Autodesk Fusion 360 part; units mm, degrees
sketch "草图1" plane through (0, 0, 0) normal (0, 0, 1) x (1, 0, 0)
  circle A0 centre (0, 0) radius 10
  circle A1 centre (0, 0) radius 7 construction
  line L0 (-4, 0) -> (3, 0)
  circle A2 centre (7, 0) radius 1.6
  circle A3 centre (0, 7) radius 1.6
  circle A4 centre (-7, 0) radius 1.6
  circle A5 centre (0, -7) radius 1.6
  dimension "d1" = 20
  dimension "d2" = 14
  dimension "d3" = 3.2
  dimension "d5" = 360
extrude "拉伸1" add sketch "草图1" along normal blind 2 makes body 1
sketch "草图2" plane through (0, 0, 2) normal (0, 0, 1) x (-1, 0, 0)
  circle A0 centre (0, 7) radius 1.6
  circle A1 centre (7, 0) radius 1.6
  circle A2 centre (-7, 0) radius 1.6
  circle A3 centre (0, -7) radius 1.6
  circle A4 centre (0, 0) radius 10
  circle A5 centre (0, 0) radius 4.5
  dimension "d8" = 9
extrude "拉伸2" add sketch "草图2" along normal blind 2.5 contours A5 bodies 1
sketch "草图3" plane through (0, 0, 4.5) normal (0, 0, 1) x (-1, 0, 0)
  circle A0 centre (0, 0) radius 4.5
  circle A1 centre (0, 0) radius 2.75
  dimension "d11" = 5.5
extrude "拉伸3" cut sketch "草图3" against normal blind 4 contours A1 bodies 1
sketch "草图4" plane through (0, 0, 0.5) normal (0, 0, 1) x (-1, 0, 0)
  circle A0 centre (0, 0) radius 2.75
  circle A1 centre (0, 0) radius 1.6
  dimension "d14" = 3.2
extrude "拉伸4" cut sketch "草图4" against normal blind 2 contours A1 bodies 1
copy_body "实体->零部件1" bodies 1 removing the originals makes body 2 in component "Component'"
component "Component'" placed x (1, 0, 0) y (0, 1, 0) z (0, 0, 1) at (0, 0, 0)
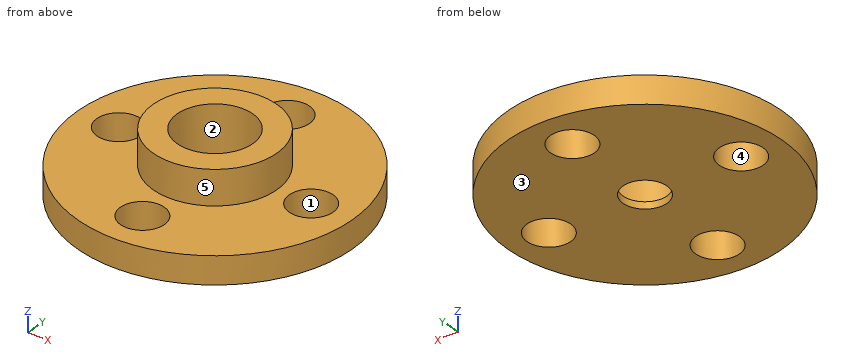
Design review of the part built by this model. Coordinates are the model's own, in mm. Face numbers are marked on the shaded views. A direction names the side the tool comes from. Give positions to 0.01 mm unless a question says otherwise; leave off trailing zeros. Order: outer loops, then holes, each group sorted by start corner. A loop starts at its lowest first (then second) coordinate and runs counter-clockwise, first axis right, second up. Notation, with made-up numbers: (45, 75) - (56, 75) arc R20 ccw to (56, 113) - close; hole circle Ø8 at (51.5, 31). An arc over 180 degrees is marked (long way). Write item = value, one per line. Start each with the question number.
Q1. To check wall thickness, follow L1, parallel to Y at x = 0, z = 0.4; L2, parallel to Y at x = 0, z = 1.2; L3, parallel to X at y = 0, z = 3.2. State the ranges of each line that lie inside material, in increasing order. Write a range as from..to.
Q2. We need section A-A on y = 0. State the section outline as (x, z) points.
Q3. Tool access review of the marked faces 1 and 2: name each direction out of +Z, -Z, +X, -X, +Y, -Y from which nothing blocks a thin tool from reaching the whole face with its end or side.
Q4. Clearance check with a flat-ended pin moving along its axis: pin 1 Ø4 at (x, y) = (7, 0) entering from +Z. State where the tip first meets the part, or that it passes through.
Q5. Mouldability with a two-part tool opening along X and no side actions: class the marked faces 3, 4 and 5 as released by +X, released by -X, zero draft, split by the parting line, or undercut.
Q6. We need section D-D on x = 7. State the section outline as (y, z) points.
Q7. We need section C-C on z = 1.05. State the section outline as (x, y) points, plus the area to 3 significant figures.
Working result:
q1.L1 = -10..-8.6, -5.4..-1.6, 1.6..5.4, 8.6..10
q1.L2 = -10..-8.6, -5.4..-2.75, 2.75..5.4, 8.6..10
q1.L3 = -4.5..-2.75, 2.75..4.5
q2.outline = (-10, 0) - (-8.6, 0) - (-8.6, 2) - (-10, 2) - close; (-5.4, 0) - (-1.6, 0) - (-1.6, 0.5) - (-2.75, 0.5) - (-2.75, 4.5) - (-4.5, 4.5) - (-4.5, 2) - (-5.4, 2) - close; (1.6, 0) - (5.4, 0) - (5.4, 2) - (4.5, 2) - (4.5, 4.5) - (2.75, 4.5) - (2.75, 0.5) - (1.6, 0.5) - close; (8.6, 0) - (10, 0) - (10, 2) - (8.6, 2) - close
q3.face_1 = +Z, -Z
q3.face_2 = +Z
q4.pin_1 = 2
q5.face_3 = zero draft
q5.face_4 = undercut
q5.face_5 = split by the parting line
q6.outline = (-7.14, 0) - (-1.6, 0) - (-1.6, 2) - (-7.14, 2) - close; (1.6, 0) - (7.14, 0) - (7.14, 2) - (1.6, 2) - close
q7.outline = circle Ø20 at (0, 0); hole circle Ø3.2 at (-7, 0); hole circle Ø5.5 at (0, 0); hole circle Ø3.2 at (0, -7); hole circle Ø3.2 at (0, 7); hole circle Ø3.2 at (7, 0)
q7.area = 258 mm²
